from build123d import *

# Parameters (mm, degrees)
SKETCH_1_R          = 13
EXTRUDE_1_DEPTH     = 8
SKETCH_2_R          = 12
CUT_EXTRUDE_1_DEPTH = 3
EXTRUDE_2_DEPTH     = 8
SKETCH_4_R          = 2.5
CUT_EXTRUDE_2_DEPTH = 2


with BuildPart() as part:
    # 草图1 → 凸台-拉伸1 (new body)
    with BuildSketch(Plane(origin=(0, 0, 0), x_dir=(1, 0, 0), z_dir=(0, 1, 0))):
        with Locations(Location((0, 0, 0), (0, 0, 270))):
            Circle(SKETCH_1_R)
    extrude(amount=EXTRUDE_1_DEPTH)

    # 草图2 → 切除-拉伸1 (cut)
    with BuildSketch(Plane(origin=(0, 8, 0), x_dir=(1, 0, 0), z_dir=(0, 1, 0))):
        with Locations(Location((0, 0, 0), (0, 0, 270))):
            Circle(SKETCH_2_R)
    extrude(amount=-CUT_EXTRUDE_1_DEPTH, mode=Mode.SUBTRACT)

    # 草图3 → 凸台-拉伸2 (add, through all)
    with BuildSketch(Plane(origin=(0, 8, 0), x_dir=(1, 0, 0), z_dir=(0, 1, 0))):
        Polygon((-12.123665589, 4.692199131), (-11.044603538, 4.692199131), (-11.653830585, 5.760922904), (-12.732892635, 5.760922904), align=None)
        Polygon((-11.124688039, 6.726166519), (-10.062019365, 6.53878936), (-10.476408948, 7.697067984), (-11.539077622, 7.884445143), align=None)
        Polygon((-9.787692472, 8.555762741), (-8.773705825, 8.186701784), (-8.980666927, 9.399341549), (-9.994653573, 9.768402506), align=None)
        Polygon((-8.153302822, 10.125396442), (-7.218807673, 9.585865416), (-7.212051886, 10.816020876), (-8.146547034, 11.355551902), align=None)
        Polygon((-6.271179191, 11.387375095), (-5.444569703, 10.693767379), (-5.224302297, 11.904060883), (-6.050911785, 12.597668599), align=None)
        Polygon((-4.198508954, 12.303354118), (-3.504901238, 11.47674463), (-3.077814927, 12.630402023), (-3.771422644, 13.457011511), align=None)
        Polygon((-1.998269147, 12.845501953), (-1.458738122, 11.911006804), (-0.837809708, 12.97297479), (-1.377340734, 13.907469938), align=None)
        Polygon((0.262687056, 12.99734571), (0.631748014, 11.983359064), (1.427651935, 12.921370282), (1.058590978, 13.935356928), align=None)
        Polygon((2.515661647, 12.754271695), (2.703038805, 11.691603022), (3.649735097, 12.477156476), (3.462357938, 13.53982515), align=None)
        Polygon((4.692199131, 12.123665589), (4.692199131, 11.044603538), (5.760922904, 11.653830585), (5.760922904, 12.732892635), align=None)
        Polygon((6.726166519, 11.124688039), (6.53878936, 10.062019365), (7.697067984, 10.476408948), (7.884445143, 11.539077622), align=None)
        Polygon((8.555762741, 9.787692472), (8.186701784, 8.773705825), (9.399341549, 8.980666927), (9.768402506, 9.994653573), align=None)
        Polygon((10.125396442, 8.153302822), (9.585865416, 7.218807673), (10.816020876, 7.212051886), (11.355551902, 8.146547034), align=None)
        Polygon((11.387375095, 6.271179191), (10.693767379, 5.444569703), (11.904060883, 5.224302297), (12.597668599, 6.050911785), align=None)
        Polygon((12.303354118, 4.198508954), (11.47674463, 3.504901238), (12.630402023, 3.077814927), (13.457011511, 3.771422644), align=None)
        Polygon((12.845501953, 1.998269147), (11.911006804, 1.458738122), (12.97297479, 0.837809708), (13.907469938, 1.377340734), align=None)
        Polygon((12.99734571, -0.262687056), (11.983359064, -0.631748014), (12.921370282, -1.427651935), (13.935356928, -1.058590978), align=None)
        Polygon((12.754271695, -2.515661647), (11.691603022, -2.703038805), (12.477156476, -3.649735097), (13.53982515, -3.462357938), align=None)
        Polygon((12.123665589, -4.692199131), (11.044603538, -4.692199131), (11.653830585, -5.760922904), (12.732892635, -5.760922904), align=None)
        Polygon((11.124688039, -6.726166519), (10.062019365, -6.53878936), (10.476408948, -7.697067984), (11.539077622, -7.884445143), align=None)
        Polygon((9.787692472, -8.555762741), (8.773705825, -8.186701784), (8.980666927, -9.399341549), (9.994653573, -9.768402506), align=None)
        Polygon((8.153302822, -10.125396442), (7.218807673, -9.585865416), (7.212051886, -10.816020876), (8.146547034, -11.355551902), align=None)
        Polygon((6.271179191, -11.387375095), (5.444569703, -10.693767379), (5.224302297, -11.904060883), (6.050911785, -12.597668599), align=None)
        Polygon((4.198508954, -12.303354118), (3.504901238, -11.47674463), (3.077814927, -12.630402023), (3.771422644, -13.457011511), align=None)
        Polygon((1.998269147, -12.845501953), (1.458738122, -11.911006804), (0.837809708, -12.97297479), (1.377340734, -13.907469938), align=None)
        Polygon((-0.262687056, -12.99734571), (-0.631748014, -11.983359064), (-1.427651935, -12.921370282), (-1.058590978, -13.935356928), align=None)
        Polygon((-2.515661647, -12.754271695), (-2.703038805, -11.691603022), (-3.649735097, -12.477156476), (-3.462357938, -13.53982515), align=None)
        Polygon((-4.692199131, -12.123665589), (-4.692199131, -11.044603538), (-5.760922904, -11.653830585), (-5.760922904, -12.732892635), align=None)
        Polygon((-6.726166519, -11.124688039), (-6.53878936, -10.062019365), (-7.697067984, -10.476408948), (-7.884445143, -11.539077622), align=None)
        Polygon((-8.555762741, -9.787692472), (-8.186701784, -8.773705825), (-9.399341549, -8.980666927), (-9.768402506, -9.994653573), align=None)
        Polygon((-10.125396442, -8.153302822), (-9.585865416, -7.218807673), (-10.816020876, -7.212051886), (-11.355551902, -8.146547034), align=None)
        Polygon((-11.387375095, -6.271179191), (-10.693767379, -5.444569703), (-11.904060883, -5.224302297), (-12.597668599, -6.050911785), align=None)
        Polygon((-12.303354118, -4.198508954), (-11.47674463, -3.504901238), (-12.630402023, -3.077814927), (-13.457011511, -3.771422644), align=None)
        Polygon((-12.845501953, -1.998269147), (-11.911006804, -1.458738122), (-12.97297479, -0.837809708), (-13.907469938, -1.377340734), align=None)
        Polygon((-12.99734571, 0.262687056), (-11.983359064, 0.631748014), (-12.921370282, 1.427651935), (-13.935356928, 1.058590978), align=None)
        Polygon((-12.754271695, 2.515661647), (-11.691603022, 2.703038805), (-12.477156476, 3.649735097), (-13.53982515, 3.462357938), align=None)
    extrude(amount=-EXTRUDE_2_DEPTH)

    # 草图4 → 切除-拉伸2 (cut)
    with BuildSketch(Plane(origin=(0, 5, 0), x_dir=(1, 0, 0), z_dir=(0, 1, 0))):
        with Locations(Location((0, 0, 0), (0, 0, 270))):
            Circle(SKETCH_4_R)
    extrude(amount=-CUT_EXTRUDE_2_DEPTH, mode=Mode.SUBTRACT)


solid = part.part
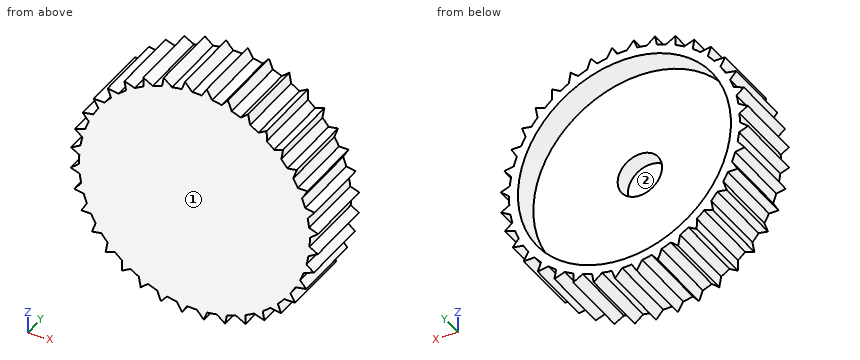
Geometry check sheet. Reference: the model listing, model coordinates, mm. Face numbers are marked on the shaded views. Coordinates: 2 decimals unless noted, no trailing zeros. Use a Markdown table: item, result. Add a question column.
1. Mould release check, pull along Z, two halves, no side actions. Record for the marked faces 1 and 2: pulls with the +Z half, pulls with the -Z half, needs draft (parallel to the pull), parting line crosses it, or undercut.
2. Go/stop test with flat-tipped pins: pin 1 Ø4 at (x, y) = (-6, 6) entering from +Z; pin 2 Ø3 at (x, z) = (-5, 2) entering from +Y; pin 3 Ø4 at (y, z) = (3, -4) entering from -X. Record where each tip stops, or that it passes through.
3. Material ranges on L1, parallel to X at y = 7, z = 0; L2, parallel to Y at x = 4.75, z = -8; L3, parallel to Z at x = 10.5, y = 4.5, recorded low to high.
Filled sheet:
| question | item | result |
|---|---|---|
| 1 | face 1 | needs draft |
| 1 | face 2 | undercut |
| 2 | pin 1 | z = 12.73 |
| 2 | pin 2 | y = 5 |
| 2 | pin 3 | x = -13.54 |
| 3 | L1 | -13 to -12, 12 to 13 |
| 3 | L2 | 0 to 5 |
| 3 | L3 | -8.15 to 7.7 |
